from build123d import *

# Parameters (mm, degrees)
BOSS_EXTRUDE1_DEPTH = 16
SHELL1_T            = -2
SKETCH2_R           = 6
BOSS_EXTRUDE2_DEPTH = 5
SKETCH4_W           = 30
SKETCH4_H           = 12
BOSS_EXTRUDE3_DEPTH = 2.5
SKETCH5_R           = 6
BOSS_EXTRUDE4_DEPTH = 5


with BuildPart() as part:
    # Sketch1 → Boss-Extrude1 (new body)
    with BuildSketch(Plane(origin=(0, 0, 0), x_dir=(1, 0, 0), z_dir=(0, 1, 0))):
        Polygon((-350, 31.008229654), (-320, 22.514402641), (-320, 61.008229654), (-350, 61.008229654), align=None)
    extrude(amount=BOSS_EXTRUDE1_DEPTH)

    # Shell1
    shell1_openings = [part.faces().sort_by_distance(p)[0] for p in [
        (-320, 8, -41.761316148),
    ]]
    offset(amount=SHELL1_T, openings=shell1_openings, kind=Kind.INTERSECTION)



with BuildPart() as body_2:
    # Sketch2 → Boss-Extrude2 (new body)
    with BuildSketch(Plane(origin=(0, 23, 0), x_dir=(1, 0, 0), z_dir=(0, 1, 0))):
        with BuildLine():
            Line((-350, 61.008229654), (-368, 61.008229654))
            ThreePointArc((-368, 61.008229654), (-383, 46.008229654), (-368, 31.008229654))
            Line((-368, 31.008229654), (-350, 31.008229654))
            Line((-350, 31.008229654), (-350, 61.008229654))
        make_face()
        with Locations((-368, 46.008229654)):
            Circle(SKETCH2_R, mode=Mode.SUBTRACT)
    extrude(amount=BOSS_EXTRUDE2_DEPTH)


with BuildPart() as part_1:
    add(part.part)

    add(body_2.part)  # Boss-Extrude3 merges body 2
    # Sketch4 → Boss-Extrude3 (add)
    with BuildSketch(Plane.ZY.offset(350)):
        with Locations((-46.008229654, 22)):
            Rectangle(SKETCH4_W, SKETCH4_H)
    boss_extrude3 = extrude(amount=-BOSS_EXTRUDE3_DEPTH)

    # Mirror14: Boss-Extrude3 across plane
    add(boss_extrude3.mirror(Plane(origin=(0, 8, 0), x_dir=(0, 0, 1), z_dir=(0, -1, 0))))

    # Sketch5 → Boss-Extrude4 (add)
    with BuildSketch(Plane.XZ.offset(12)):
        with BuildLine():
            Line((-350, -61.008229654), (-350, -31.008229654))
            Line((-350, -31.008229654), (-368, -31.008229654))
            ThreePointArc((-368, -31.008229654), (-383, -46.008229654), (-368, -61.008229654))
            Line((-368, -61.008229654), (-350, -61.008229654))
        make_face()
        with Locations((-368, -46.008229654)):
            Circle(SKETCH5_R, mode=Mode.SUBTRACT)
    extrude(amount=-BOSS_EXTRUDE4_DEPTH)


solid = part_1.part
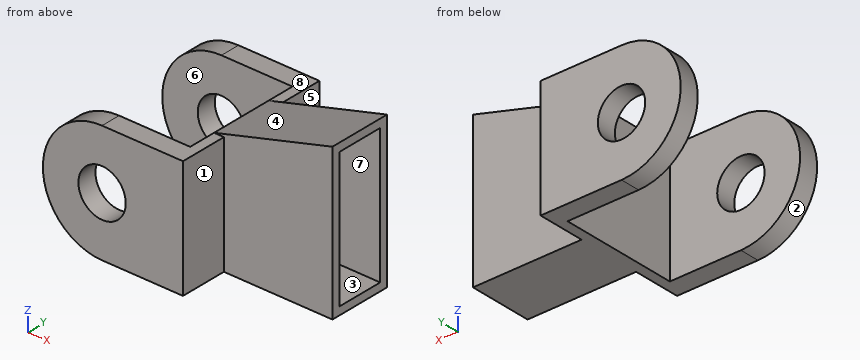
Geometry: final body of the model. Coordinates: model frame, mm. Face numbers are marked on the shaded views. A direction names the side the tool comes from. Give positions to 0.01 mm unless a question says otherwise; leave off trailing zeros. Order: outer loops, then holes, each group sorted by start corner. A loop starts at its lowest first (then second) coordinate and runs counter-clockwise, first axis right, second up. Notation, with made-up numbers: (88.5, 53) -> (131.5, 53) arc R22 ccw to (131.5, 82) -> close; hole circle Ø3 at (10.25, 52.5). An arc over 180 degrees is marked (long way). Write each question's results on one line, items separated by ' | '.
1) Cut plane B-B (z = -47). Output: boundary loops of the cut face in (x, y), and give its area (3 significant figures).
Geometry says:
outline: (-382.97, -12) -> (-373.92, -12) -> (-373.92, -7) -> (-382.97, -7) -> close; (-382.97, 23) -> (-373.92, 23) -> (-373.92, 28) -> (-382.97, 28) -> close; (-362.08, -12) -> (-347.5, -12) -> (-347.5, 0) -> (-320, 0) -> (-320, 2) -> (-348, 2) -> (-348, 14) -> (-320, 14) -> (-320, 16) -> (-347.5, 16) -> (-347.5, 28) -> (-362.08, 28) -> (-362.08, 23) -> (-350, 23) -> (-350, -7) -> (-362.08, -7) -> close | area: 415 mm²
2) First-contact query: pin 1 Ø13 at (y, z) = (10.5, -50.5) entering from +X; pin 2 Ø9.5 at (x, y) = (-354, 24) entering from +Z; pin 3 Ø3 at (y, z) = (7.5, -44) entering from +X; pin 4 Ø13 at (x, y) = (-340, 6.5) entering from +Z. Flat tips, straight axial feed; report the tip coordinate or a pass-through.
Geometry says:
pin 1: stops at x = -320 | pin 2: stops at z = -31.01 | pin 3: stops at x = -348 | pin 4: stops at z = -26.34
3) Cut plane D-D (y = 25). Output: boundary loops of the cut face in (x, z).
Geometry says:
outline: (-368, -61.01) -> (-347.5, -61.01) -> (-347.5, -31.01) -> (-368, -31.01) arc R15 ccw to start; hole circle Ø12 at (-368, -46.01)
4) Line query: line 1 along Y through (x, z) = (-332.5, -53); line 2 along Z through (x, y) = (-368, 26); line 3 along Y through (x, z) = (-352, -36.5). Output: solid intervals per line, ascending.
Geometry says:
line 1: y = 0 to 2, 14 to 16 | line 2: z = -61.01 to -52.01, -40.01 to -31.01 | line 3: y = -12 to -7, 23 to 28
5) Cut plane C-C (x = -333.5). Output: boundary loops of the cut face in (y, z).
Geometry says:
outline: (0, -61.01) -> (16, -61.01) -> (16, -26.34) -> (0, -26.34) -> close; hole (2, -59.01) -> (14, -59.01) -> (14, -28.42) -> (2, -28.42) -> close
6) Cut plane A-A (y = 7). Output: boundary loops of the cut face in (x, z).
Geometry says:
outline: (-350, -61.01) -> (-320, -61.01) -> (-320, -59.01) -> (-348, -59.01) -> (-348, -32.52) -> (-320, -24.59) -> (-320, -22.51) -> (-350, -31.01) -> close
7) Draft query along Z for the marked faces 1, 2 and 3. Return one class per face: released by +Z, released by -Z, zero draft, split by the parting line, or undercut.
Geometry says:
face 1: zero draft | face 2: split by the parting line | face 3: undercut
8) Set-up query: the marked faces 4, 5, 6, 7 and 8. Return all of +Z, -Z, +X, -X, +Y, -Y with unobstructed straight access to the full face (end or side cutting, diameter ignored); none if empty.
Geometry says:
face 4: +Z, -X, +Y, -Y | face 5: +Z, -Z, +X, +Y | face 6: +Z, -Z, -X | face 7: +X | face 8: +Z, +X, -X, +Y
